Job drawing, mm, ordinate dimensions from the low corner. One solid piece. Round coordinates to 2 decimals unless told otherwise and drop trailing zeros. Write each loop counter-clockwise with the first axis right and the second up, starting at its lowest first coordinate (ties: lowest second). Pieces come first, ordered by that corner, then holes. Notation, with made-up numbers: (3.5, 8) - (39.5, 8) arc R25 cw to (39.5, 27) - close; hole circle Ø7 at (3.25, 58.25). An arc over 180 degrees is marked (long way). Write each question's results on one line, items separated by ' | '.
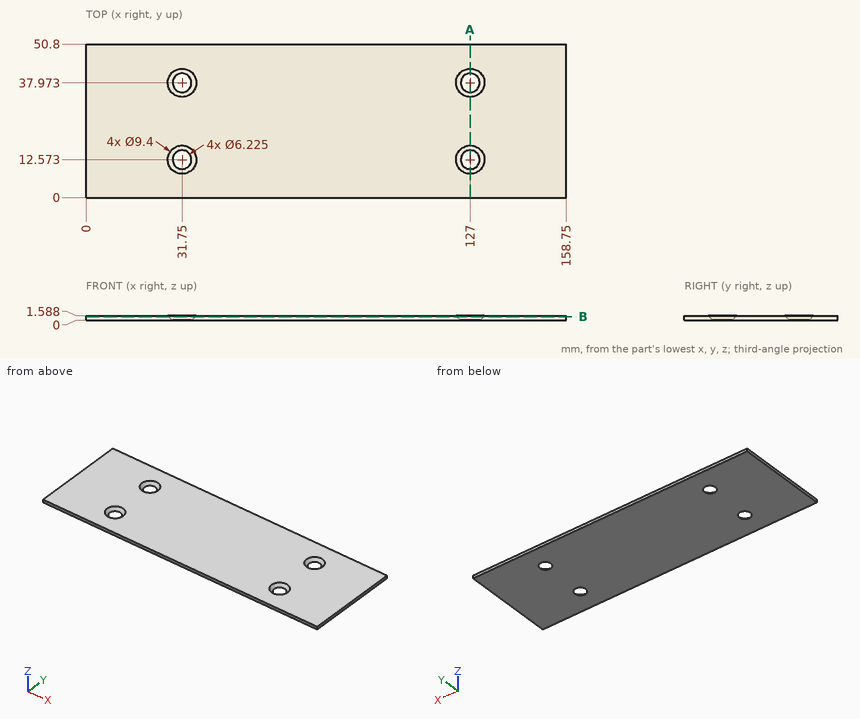
(1) Slice it at A-A, the plane x = 127. Write the cut outline in (y, z) (1 decimal).
Worked answers:
outline: (0, 0) - (9.5, 0) - (7.9, 1.6) - (0, 1.6) - close; (15.7, 0) - (34.9, 0) - (33.3, 1.6) - (17.3, 1.6) - close; (41.1, 0) - (50.8, 0) - (50.8, 1.6) - (42.7, 1.6) - close
(2) Drill centre lines: probe 1 along X at (y, z) = (15, 0.35); probe 2 along Y at (x, z) = (124.5, 0.25) (1 decimal); probe 3 along X at (y, z) = (14, 0.9). Where is each one in solid material? Low to high. Write a range as [from, to].
Worked answers:
probe 1: x = [0, 29.28], [34.22, 124.53], [129.47, 158.75] | probe 2: y = [0, 10.3], [14.8, 35.7], [40.2, 50.8] | probe 3: x = [0, 28], [35.5, 123.25], [130.75, 158.75]
(3) Slice it at B-B, the plane z = 1.3. State how many separate pieces and enclosed holes the cut face has, and give its area (3 significant figures).
Worked answers:
separate pieces: 1 | enclosed holes: 4 | area: 7,820 mm2
